Work out the finished part from the listing and answer in its coordinate system (mm). A direction names the side the tool comes from. Give positions to 0.01 mm unless a question says otherwise; leave off trailing zeros. Loops run counter-clockwise (first coordinate to the right, second up) from the corner with the lowest first, then second, coordinate; pieces in that order, holes last. Notation, with made-up numbers: (41.25, 30.5) - (81.25, 30.5) arc R23 cw to (81.25, 67.5) - close; hole circle Ø8 at (57.25, 87.5). An arc over 180 degrees is marked (long way). One line per question, with ' | ' between items.
from build123d import *

# Parameters (mm, degrees)
BOX_W        = 18
BOX_H        = 100
BOX_DEPTH    = 80
SKETCH001_W  = 144
SKETCH001_H  = 154
PAD_DEPTH    = 15
SKETCH002_W  = 114
SKETCH002_H  = 124
PAD002_DEPTH = 5
SKETCH_R     = 4
PAD001_DEPTH = 160


with BuildPart() as cube:
    # Box → Box (new body)
    with BuildSketch(Plane(origin=(-91.5, -41, 20), x_dir=(1, 0, 0), z_dir=(0, 0, 1))):
        with Locations((9, 50)):
            Rectangle(BOX_W, BOX_H)
    extrude(amount=BOX_DEPTH)


with BuildPart() as baseframe:
    # Sketch001 → Pad (new body)
    with BuildSketch(Plane.XY.offset(20)):
        with Locations((-1.5, 9)):
            Rectangle(SKETCH001_W, SKETCH001_H)
    extrude(amount=-PAD_DEPTH)


with BuildPart() as cutblock:
    # Sketch002 → Pad002 (new body)
    with BuildSketch(Plane.XY.offset(5)):
        with Locations((-1.5, 9)):
            Rectangle(SKETCH002_W, SKETCH002_H)
    extrude(amount=-PAD002_DEPTH)

    # Fusion: union BaseFrame
    add(baseframe.part)


with BuildPart() as cut001:
    # Sketch → Pad001 (new body)
    with BuildSketch(Plane(origin=(0, -71, 20), x_dir=(1, 0, 0), z_dir=(0, -1, 0))):
        with BuildLine():
            Line((-91.5, -20), (-91.5, 71.000001))
            ThreePointArc((-73.5, 71), (-82.5, 80), (-91.5, 71.000001))
            Line((-73.5, 0), (-73.5, 71))
            Line((73.5, 0), (-73.5, 0))
            Line((73.5, -20), (73.5, 0))
            Line((-91.5, -20), (73.5, -20))
        make_face()
        with Locations((-82.5, 71)):
            Circle(SKETCH_R, mode=Mode.SUBTRACT)
        with Locations((-82.5, 11)):
            Circle(SKETCH_R, mode=Mode.SUBTRACT)
    extrude(amount=-PAD001_DEPTH)

    # Cut: cut CutBlock
    add(cutblock.part, mode=Mode.SUBTRACT)

    # Cut001: cut Cube
    add(cube.part, mode=Mode.SUBTRACT)


solid = cut001.part
1. Determine the mould class of faces 1 (the flat face through (-73.5, 8, 19)), 2 (the flat face through (-27, 89, 17)), 3 (the flat face through (71, -27, 20)) for opening direction Y: +Y half, -Y half, draft (parallel to the pull), parting line (faces both ways), or undercut.
Evaluation:
face 1: undercut | face 2: +Y half | face 3: draft
2. Find section D-D on x = -82.5. Write down the section's boundary in (y, z), then the cut area to 3 significant figures.
Evaluation:
outline: (-71, 0) - (89, 0) - (89, 27) - (59, 27) - (59, 20) - (-41, 20) - (-41, 27) - (-71, 27) - close; (-71, 35) - (-41, 35) - (-41, 87) - (-71, 87) - close; (-71, 95) - (-41, 95) - (-41, 100) - (-71, 100) - close; (59, 35) - (89, 35) - (89, 87) - (59, 87) - close; (59, 95) - (89, 95) - (89, 100) - (59, 100) - close | area: 7,040 mm2
3. Find section C-C on y = 79. Write down the section's boundary in (x, z).
Evaluation:
outline: (-91.5, 0) - (73.5, 0) - (73.5, 20) - (70.5, 20) - (70.5, 5) - (-73.5, 5) - (-73.5, 91) arc R9 ccw to (-91.5, 91) - close; hole circle Ø8 at (-82.5, 31); hole circle Ø8 at (-82.5, 91)
4. Consider L1, parallel to Z at x = -82.5, y = -57; L2, parallel to Y at x = 29, z = 13; L3, parallel to X at y = 11, z = 10. Determine where each line is inside the solid, lowest interval first.
Evaluation:
L1: 0 to 27, 35 to 87, 95 to 100 | L2: -71 to -68, 86 to 89 | L3: -91.5 to -73.5, 70.5 to 73.5
5. Which of the six approach directions +Z, -Z, +X, -X, +Y, -Y give full straight-line access (tool end or side, diameter ignored) to faces 4 (the flat face through (-83, 59, 59)), 5 (the flat face through (-67, 10, 5)), 6 (the flat face through (-65, 8, 0)), 7 (the flat face through (73.5, 8, 10)), 8 (the flat face through (-58.5, 8, 3))?
Evaluation:
face 4: +Z, +X, -X | face 5: +Z | face 6: -Z, +X, -X, +Y, -Y | face 7: +Z, -Z, +X, +Y, -Y | face 8: +Z, -Z
6. Find section A-A on z = 31. Write down the section's boundary in (x, y), then the cut area to 3 significant figures.
Evaluation:
outline: (-91.5, -71) - (-86.5, -71) - (-86.5, -41) - (-91.5, -41) - close; (-91.5, 59) - (-86.5, 59) - (-86.5, 89) - (-91.5, 89) - close; (-78.5, -71) - (-73.5, -71) - (-73.5, -41) - (-78.5, -41) - close; (-78.5, 59) - (-73.5, 59) - (-73.5, 89) - (-78.5, 89) - close | area: 600 mm2
7. Flat-ended cylindrical pins translate along their axes: pin 1 (20 mm diameter, centred on x = -80.5, y = 21, fed in from +Z); pin 2 (2 mm diameter, centred on x = -48, z = 21.5, fed in from -Y). Find the tip coordinate at first contact, or state that the pin passes through.
Evaluation:
pin 1: z = 20 | pin 2: through
8. Find section B-B on x = 11.5. Write down the section's boundary in (y, z), then the cut area to 3 significant figures.
Evaluation:
outline: (-71, 0) - (-53, 0) - (-53, 5) - (-68, 5) - (-68, 20) - (-71, 20) - close; (71, 0) - (89, 0) - (89, 20) - (86, 20) - (86, 5) - (71, 5) - close | area: 270 mm2
